from build123d import *

# Parameters (mm, degrees)
SKETCH1_R           = 20
BOSS_EXTRUDE1_DEPTH = 55
SHELL1_T            = -1
FILLET1_R           = 2
FILLET7_R           = 1


with BuildPart() as part:
    # Sketch1 → Boss-Extrude1 (new body)
    with BuildSketch(Plane(origin=(0, 0, 0), x_dir=(1, 0, 0), z_dir=(0, 1, 0))):
        with Locations(Location((0, 0, 0), (0, 0, 270))):
            Circle(SKETCH1_R)
    extrude(amount=BOSS_EXTRUDE1_DEPTH)

    # Shell1
    shell1_openings = [part.faces().sort_by_distance(p)[0] for p in [
        (0, 55, 0),
    ]]
    offset(amount=SHELL1_T, openings=shell1_openings, kind=Kind.INTERSECTION)

    # Fillet1
    fillet1_edges = [part.edges().sort_by_distance(p)[0] for p in [
        (0, 0, -20),
    ]]
    fillet(fillet1_edges, radius=FILLET1_R)

    # Fillet7
    fillet7_edges = [part.edges().sort_by_distance(p)[0] for p in [
        (0, 55, -20),
    ]]
    fillet(fillet7_edges, radius=FILLET7_R - 0.0001)  # a hair under: the kernel refuses the full size


solid = part.part
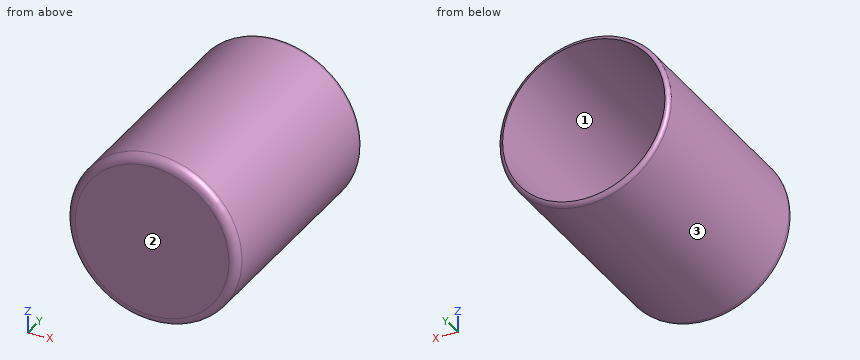
Source: CAD feature listing. Evaluate the final solid. Frame: model axes, mm. Face numbers are marked on the shaded views. Coordinates: 2 decimals unless noted, no trailing zeros. Write each loop counter-clockwise with the first axis right and the second up, starting at its lowest first coordinate (ties: lowest second). Pieces come first, ordered by that corner, then holes. Notation, with made-up numbers: M -30,26.5 L 5,26.5 A21 cw 5,57.5 Z; hole C 55.5,49 d1. An arc over 180 degrees is marked long. Use a Markdown table: item, result.
1) Ray query, L1, parallel to X at y = 20, z = 0; L2, parallel to Y at x = 6.5, z = 14; L3, parallel to Z at x = 16, y = 26. Return the intervals inside material, ascending.
Conclusion:
| item | result |
|---|---|
| L1 | x = -20 to -19, 19 to 20 |
| L2 | y = 0 to 1 |
| L3 | z = -12 to -10.25, 10.25 to 12 |
2) First-contact query: pin 1 Ø4 at (y, z) = (28, -0.5) entering from -X; pin 2 Ø2 at (y, z) = (24.5, 15) entering from +X; pin 3 Ø19 at (x, z) = (-2.5, 3.5) entering from +Y. Flat tips, straight axial feed; report the tip coordinate or a pass-through.
Conclusion:
| item | result |
|---|---|
| pin 1 | stops at x = -20 |
| pin 2 | stops at x = 14.28 |
| pin 3 | stops at y = 1 |
3) Mould query, pull axis X, two halves, no side actions, for the marked faces 1, 2 and 3. Classes: pulls with the +X half, pulls with the -X half, needs draft (parallel to the pull), parting line crosses it, or undercut.
Conclusion:
| item | result |
|---|---|
| face 1 | undercut |
| face 2 | needs draft |
| face 3 | parting line crosses it |
4) Section C-C, the plane y = 44.5. Output: boundary loops of the cut face in (x, z).
Conclusion:
| item | result |
|---|---|
| outline | C 0,0 d40; hole C 0,0 d38 |
